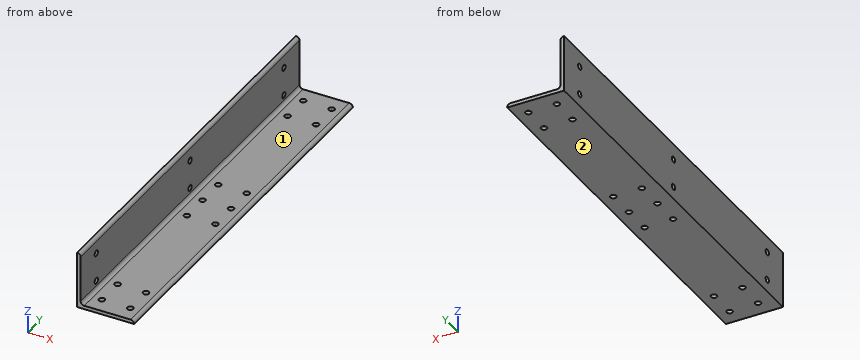
```python
from build123d import *

# Parameters (mm, degrees)
F1_DEPTH = 355.6
F2_R     = 2.6162
F3_DEPTH = 3.176
F4_R     = 2.6162
F5_DEPTH = 3.176


with BuildPart() as f1:
    # F0 (on Front) → F1 (new body)
    with BuildSketch(Plane.XZ):
        with BuildLine():
            Line((-50.8, 0), (0, 0))
            ThreePointArc((0, 0), (-0.929936, 2.245064), (-3.175, 3.175))
            Line((-3.175, 3.175), (-44.45, 3.175))
            ThreePointArc((-44.45, 3.175), (-46.695064, 4.104936), (-47.625, 6.35))
            Line((-47.625, 6.35), (-47.625, 47.625))
            ThreePointArc((-47.625, 47.625), (-48.554936, 49.870064), (-50.8, 50.8))
            Line((-50.8, 50.8), (-50.8, 0))
        make_face()
    extrude(amount=F1_DEPTH)

    # F2 (on face) → F3 (cut, through all)
    with BuildSketch(Plane.YZ.offset(-47.625)):
        with Locations((-330.2, 11.1125)):
            Circle(F2_R)
        with Locations((-177.8, 11.1125)):
            Circle(F2_R)
        with Locations((-25.4, 11.1125)):
            Circle(F2_R)
        with Locations((-330.2, 36.5125)):
            Circle(F2_R)
        with Locations((-177.8, 36.5125)):
            Circle(F2_R)
        with Locations((-25.4, 36.5125)):
            Circle(F2_R)
    extrude(amount=-F3_DEPTH, mode=Mode.SUBTRACT)

    # F4 (on face) → F5 (cut, through all)
    with BuildSketch(Plane.XY.offset(3.175)):
        with Locations((-36.5125, -341.3125)):
            Circle(F4_R)
        with Locations((-36.5125, -14.2875)):
            Circle(F4_R)
        with Locations((-36.5125, -177.8)):
            Circle(F4_R)
        with Locations((-11.1125, -341.3125)):
            Circle(F4_R)
        with Locations((-11.1125, -177.8)):
            Circle(F4_R)
        with Locations((-11.1125, -14.2875)):
            Circle(F4_R)
        with Locations((-36.5125, -203.2)):
            Circle(F4_R)
        with Locations((-11.1125, -203.2)):
            Circle(F4_R)
        with Locations((-36.5125, -152.4)):
            Circle(F4_R)
        with Locations((-11.1125, -152.4)):
            Circle(F4_R)
        with Locations((-11.1125, -39.6875)):
            Circle(F4_R)
        with Locations((-36.5125, -39.6875)):
            Circle(F4_R)
        with Locations((-11.1125, -315.9125)):
            Circle(F4_R)
        with Locations((-36.5125, -315.9125)):
            Circle(F4_R)
    extrude(amount=-F5_DEPTH, mode=Mode.SUBTRACT)


solid = f1.part
```
Work out the finished part from the listing and answer in its coordinate system (mm). Face numbers are marked on the shaded views. A direction names the side the tool comes from. Give positions to 0.01 mm unless a question says otherwise; leave off trailing zeros. Order: outer loops, then holes, each group sorted by start corner. A loop starts at its lowest first (then second) coordinate and runs counter-clockwise, first axis right, second up. Notation, with made-up numbers: (60.25, 50.5) - (110.25, 50.5) arc R16 cw to (110.25, 66.5) - close; hole circle Ø8 at (-8, 74). An arc over 180 degrees is marked (long way). One line per item, written item: value. Start each with the question number.
1. Section A-A, the plane y = -61.5 is taken. Write down the section's boundary in (x, z) (3 decimals), then the cut area to 3 significant figures.
2. Consider line 1 (X direction, y = -203.2, z = 0.9); line 2 (X direction, y = -152.4, z = 1.85); line 3 (X direction, y = -162, z = 33) (3 decimals). Determine where each line is inside the solid, lowest interval first.
3. Section B-B, the plane z = 27 is taken. Write down the section's boundary in (x, y) (3 decimals), then the cut area to 3 significant figures.
4. Which of the six approach directions +Z, -Z, +X, -X, +Y, -Y give full straight-line access (tool end or side, diameter ignored) to the marked faces 1 and 2?
5. Each of these flat-tipped pins is pushed along its axis until it touches: pin 1 Ø2 at (y, z) = (-296, 26) entering from +X (3 decimals); pin 2 Ø7 at (x, y) = (-36.51, -152.4) entering from +Z (3 decimals). Where does it stop, or does it pass through?
Filled sheet:
1. outline: (-50.8, 0) - (0, 0) arc R3.175 ccw to (-3.175, 3.175) - (-44.45, 3.175) arc R3.175 cw to (-47.625, 6.35) - (-47.625, 47.625) arc R3.175 ccw to (-50.8, 50.8) - close
1. area: 310 mm²
2. line 1: -50.8 to -39.13, -33.9 to -13.73, -8.5 to -0.13
2. line 2: -50.8 to -39.13, -33.9 to -13.73, -8.5 to -0.59
2. line 3: -50.8 to -47.625
3. outline: (-50.8, -355.6) - (-47.625, -355.6) - (-47.625, 0) - (-50.8, 0) - close
3. area: 1,130 mm²
4. face 1: +Z, +X, +Y, -Y
4. face 2: -Z, +X, -X, +Y, -Y
5. pin 1: x = -47.625
5. pin 2: z = 3.175
